For this review, take the finished solid that the model builds, in its own axes (mm). A direction names the side the tool comes from. Round coordinates to 2 decimals unless told otherwise and drop trailing zeros. Write each loop counter-clockwise with the first axis right and the second up, starting at its lowest first coordinate (ties: lowest second). Pieces come first, ordered by that corner, then holes.
from build123d import *

# Parameters (mm, degrees)
AUFSATZ_LINEAR_AUSTRAGEN1_DEPTH = 28
AUFSATZ_LINEAR_AUSTRAGEN2_DEPTH = 1.5


with BuildPart() as part:
    # Skizze2 → Aufsatz-Linear austragen1 (new body)
    with BuildSketch(Plane.XY):
        with BuildLine():
            Line((0, 0), (112, 0))
            Line((112, 0), (112, 4.782759721))
            ThreePointArc((112, 4.782759721), (110.475234931, 9.315591895), (106.520915328, 12.005356293))
            ThreePointArc((106.520915328, 12.005356293), (96.560287053, 16.884466202), (89, 25))
            Line((89, 25), (71.329947288, 46.937212002))
            ThreePointArc((71.329947288, 46.937212002), (39.188190047, 61.014465273), (9.219098516, 42.763022288))
            ThreePointArc((9.219098516, 42.763022288), (7.87025923, 39.559587955), (7.496101502, 36.103959945))
            Line((7.496101502, 36.103959945), (7.8, 28))
            Line((7.8, 28), (-0.129590409, 13.132017983))
            ThreePointArc((-0.129590409, 13.132017983), (-0.671897822, 11.455219867), (-0.598761004, 9.694424518))
            Line((-0.598761004, 9.694424518), (1, 2.5))
            Line((1, 2.5), (0, 0))
        make_face()
    extrude(amount=-AUFSATZ_LINEAR_AUSTRAGEN1_DEPTH)

    # Skizze3 → Aufsatz-Linear austragen2 (add)
    with BuildSketch(Plane.XY):
        with BuildLine():
            Line((93.075548833, 27.910970342), (75.223854733, 50.073688497))
            ThreePointArc((75.223854733, 50.073688497), (38.852918908, 66.003211935), (4.94052586, 45.350263295))
            ThreePointArc((4.94052586, 45.350263295), (3.029670204, 40.812064656), (2.499613424, 35.916591642))
            Line((2.499613424, 35.916591642), (2.752920862, 29.161726616))
            Line((2.752920862, 29.161726616), (-4.541355115, 15.48495916))
            ThreePointArc((-4.541355115, 15.48495916), (-5.625969942, 12.131362926), (-5.479696305, 8.609772229))
            Line((-5.479696305, 8.609772229), (-3.880935301, 1.415347711))
            Line((-3.880935301, 1.415347711), (1, 2.5))
            Line((1, 2.5), (-0.598761004, 9.694424518))
            ThreePointArc((-0.598761004, 9.694424518), (-0.671897822, 11.455219867), (-0.129590409, 13.132017983))
            Line((-0.129590409, 13.132017983), (7.8, 28))
            Line((7.8, 28), (7.496101502, 36.103959945))
            ThreePointArc((7.496101502, 36.103959945), (7.87025923, 39.559587955), (9.219098516, 42.763022288))
            ThreePointArc((9.219098516, 42.763022288), (39.188190047, 61.014465273), (71.329947288, 46.937212002))
            Line((71.329947288, 46.937212002), (89, 25))
            ThreePointArc((89, 25), (96.560287053, 16.884466202), (106.520915328, 12.005356293))
            ThreePointArc((106.520915328, 12.005356293), (110.475234931, 9.315591895), (112, 4.782759721))
            Line((112, 4.782759721), (112, 0))
            Line((112, 0), (117, 0))
            Line((117, 0), (117, 4.782759721))
            ThreePointArc((117, 4.782759721), (114.458724885, 12.337480011), (107.868192213, 16.820420674))
            ThreePointArc((107.868192213, 16.820420674), (99.43268373, 20.97962177), (93.075548833, 27.910970342))
        make_face()
    aufsatz_linear_austragen2 = extrude(amount=-AUFSATZ_LINEAR_AUSTRAGEN2_DEPTH)

    # Spiegeln1: Aufsatz-Linear austragen2 across plane
    add(aufsatz_linear_austragen2.mirror(Plane.XY.offset(-14)))


solid = part.part
(1) We need section D-D, the plane x = 42. Give the boundary of the cut face in (y, z).
Geometry check:
outline: (0, -28) - (66.1, -28) - (66.1, -26.5) - (61.1, -26.5) - (61.1, -1.5) - (66.1, -1.5) - (66.1, 0) - (0, 0) - close
(2) For pin 1 Ø2 at (x, z) = (98.5, -17.5) entering from -Y; pin 2 Ø2.5 at (y, z) = (1.5, -11.5) entering from +X; pin 3 Ø12 at (y, z) = (41.5, -24.5) entering from -X; pin 4 Ø2 at (y, z) = (20.5, -13) entering from -X, all flat-tipped, find the tip position at first contact; note any pin that passes through.
Geometry check:
pin 1: stops at y = 0
pin 2: stops at x = 112
pin 3: stops at x = 2.49
pin 4: stops at x = 3.27
(3) Mouldability with a two-part tool opening along Y and no side actions: class faces 1 (the face through (55, 26, 0)), 2 (the face through (0.51, 1.27, -13.8)), 3 (the face through (99.54, 20.9, -27.26)) as pulls with the +Y half, pulls with the -Y half, needs draft (parallel to the pull), parting line crosses it, or undercut.
Geometry check:
face 1: needs draft
face 2: undercut
face 3: pulls with the +Y half
(4) We need section A-A, the plane x = 98. Give the boundary of the cut face in (y, z), and give its area (3 significant figures).
Geometry check:
outline: (0, -28) - (22.14, -28) - (22.14, -26.5) - (15.88, -26.5) - (15.88, -1.5) - (22.14, -1.5) - (22.14, 0) - (0, 0) - close
area: 463 mm2
(5) We need section C-C, the plane y = 54. Give the boundary of the cut face in (x, z).
Geometry check:
outline: (11.83, -28) - (71.64, -28) - (71.64, -26.5) - (63.85, -26.5) - (63.85, -1.5) - (71.64, -1.5) - (71.64, 0) - (11.83, 0) - (11.83, -1.5) - (19.62, -1.5) - (19.62, -26.5) - (11.83, -26.5) - close
(6) For faces 4 (the face through (96.69, 16.79, -13.82)), 5 (the face through (0.2, 6.1, -13.8)), 6 (the face through (112, 2, -14)), list the 3-axis set-ups (+Z, -Z, +X, -X, +Y, -Y) from which the entire face can be reached by the end or side of a thin tool; tool diameter is ignored.
Geometry check:
face 4: +X, +Y
face 5: -X
face 6: +X, +Y, -Y
(7) We need section B-B, the plane z = -18.5. Give the boundary of the cut face in (x, y).
Geometry check:
outline: (-0.6, 9.69) - (1, 2.5) - (0, 0) - (112, 0) - (112, 4.78) arc R7.5 ccw to (106.52, 12.01) arc R30.53 cw to (89, 25) - (71.33, 46.94) arc R38 ccw to (9.22, 42.76) arc R12 ccw to (7.5, 36.1) - (7.8, 28) - (-0.13, 13.13) arc R5 ccw to start
(8) For line 1 along Z through (x, y) = (87, 31); line 2 along Y through (x, z) = (89, -26); line 3 along X through (y, z) = (42, -14.25), list the stretches that pass through material, from the lowest coordinate up.
Geometry check:
line 1: z = -28 to -26.5, -1.5 to 0
line 2: y = 0 to 25
line 3: x = 8.79 to 75.31
